Could you check a few things on this model? Use its own coordinates, in mm. Round coordinates to 2 decimals unless told otherwise and drop trailing zeros. Write each loop counter-clockwise with the first axis right and the second up, starting at its lowest first coordinate (ties: lowest second). Pieces come first, ordered by that corner, then holes. Notation, with made-up numbers: (32, 28) - (67, 28) arc R14 cw to (67, 35) - close; hole circle Ø11 at (-31, 29). An arc over 180 degrees is marked (long way). Write each question's results on one line, items separated by ' | '. Start each with the question number.
(1) Imagine slicing it at D-D on z = -28.5. Write out the boundary of the cut face in (x, y).
(2) Imagine slicing it at A-A on z = 0. Write out the boundary of the cut face in (x, y).
(3) Please list where these lines run through material, in increasing order: line 1 (X direction, y = 1.8, z = -24.5); line 2 (Z direction, x = -50, y = 2.05); line 3 (X direction, y = 1.2, z = 0). Write a range as [from, to].
(4) For P1, Ø3, axis at x = -100, z = -20, coming from the +Y side; P2, Ø0.9, axis at x = -119, y = 2, coming from the -Z side; P3, Ø1.5, axis at y = 1.5, z = -24.5, coming from the -X side, each with a flat end and sliding along its axis, tell me the tip position at first contact or that it passes through.
(5) Imagine slicing it at C-C on y = 0.65. State how many separate pieces and enclosed holes the cut face has, then the cut area to 3 significant figures.
(6) Imagine slicing it at B-B on x = 50. Write out the boundary of the cut face in (y, z).
(7) Thinking about a two-plate mould opening in X: for faces 1 (the flat face through (-2, 3, 15)), 2 (the cylindrical face through (-60, 2, 0)), 3 (the cylindrical face through (76, 1, 42)), which applies, +X half, -X half, draft (parallel to the pull), parting line (faces both ways), or undercut?
```python
from build123d import *

# Parameters (mm, degrees)
SKETCH1_W           = 220
SKETCH1_H           = 80
BOSS_EXTRUDE1_DEPTH = 3
SKETCH2_W           = 20
SKETCH2_H           = 20
SKETCH2_R           = 2
BOSS_EXTRUDE2_DEPTH = 3
FILLET1_R           = 5
SKETCH3_R           = 2
CUT_EXTRUDE1_DEPTH  = 3
SKETCH4_R           = 1.5
CUT_EXTRUDE2_DEPTH  = 3
SKETCH5_W           = 150
SKETCH5_H           = 22
BOSS_EXTRUDE3_DEPTH = 3
FILLET2_R           = 5
SKETCH6_R           = 10
CUT_EXTRUDE3_DEPTH  = 3
SKETCH7_R           = 2
CUT_EXTRUDE4_DEPTH  = 3


with BuildPart() as part:
    # Sketch1 → Boss-Extrude1 (new body)
    with BuildSketch(Plane(origin=(0, 0, 0), x_dir=(1, 0, 0), z_dir=(0, 1, 0))):
        Rectangle(SKETCH1_W, SKETCH1_H)
    extrude(amount=BOSS_EXTRUDE1_DEPTH)

    # Sketch2 → Boss-Extrude2 (add)
    with BuildSketch(Plane(origin=(0, 3, 0), x_dir=(1, 0, 0), z_dir=(0, 1, 0))):
        with Locations((-120, -30)):
            Rectangle(SKETCH2_W, SKETCH2_H)
        with Locations((-120, -32.5)):
            Circle(SKETCH2_R, mode=Mode.SUBTRACT)
    boss_extrude2 = extrude(amount=-BOSS_EXTRUDE2_DEPTH)

    # Mirror1: Boss-Extrude2 across plane
    add(boss_extrude2.mirror(Plane(origin=(0, 0, 0), x_dir=(0, 0, 1), z_dir=(1, 0, 0))))

    # Fillet1
    fillet1_edges = [part.edges().sort_by_distance(p)[0] for p in [
        (-110, 1.5, 20),
        (110, 1.5, 20),
    ]]
    fillet(fillet1_edges, radius=FILLET1_R)

    # Sketch3 → Cut-Extrude1 (cut)
    with BuildSketch(Plane(origin=(0, 3, 0), x_dir=(1, 0, 0), z_dir=(0, 1, 0))):
        with Locations((-100, 20)):
            Circle(SKETCH3_R)
        with Locations((100, 20)):
            Circle(SKETCH3_R)
    extrude(amount=-CUT_EXTRUDE1_DEPTH, mode=Mode.SUBTRACT)

    # Sketch4 → Cut-Extrude2 (cut)
    with BuildSketch(Plane(origin=(0, 3, 0), x_dir=(1, 0, 0), z_dir=(0, 1, 0))):
        with Locations((0, 24.5)):
            Circle(SKETCH4_R)
        with Locations((58, 24.5)):
            Circle(SKETCH4_R)
        with Locations((58, -24.5)):
            Circle(SKETCH4_R)
        with Locations((0, -24.5)):
            Circle(SKETCH4_R)
    extrude(amount=-CUT_EXTRUDE2_DEPTH, mode=Mode.SUBTRACT)

    # Sketch5 → Boss-Extrude3 (add)
    with BuildSketch(Plane(origin=(0, 3, 0), x_dir=(1, 0, 0), z_dir=(0, 1, 0))):
        with Locations((0, -40)):
            Rectangle(SKETCH5_W, SKETCH5_H)
    extrude(amount=-BOSS_EXTRUDE3_DEPTH)

    # Fillet2
    fillet2_edges = [part.edges().sort_by_distance(p)[0] for p in [
        (-75, 1.5, 40),
        (75, 1.5, 40),
    ]]
    fillet(fillet2_edges, radius=FILLET2_R)

    # Sketch6 → Cut-Extrude3 (cut)
    with BuildSketch(Plane(origin=(0, 3, 0), x_dir=(1, 0, 0), z_dir=(0, 1, 0))):
        with Locations((-50, 0)):
            Circle(SKETCH6_R)
        Circle(SKETCH6_R)
        with Locations((50, 0)):
            Circle(SKETCH6_R)
    extrude(amount=-CUT_EXTRUDE3_DEPTH, mode=Mode.SUBTRACT)

    # Sketch7 → Cut-Extrude4 (cut)
    with BuildSketch(Plane(origin=(0, 3, 0), x_dir=(1, 0, 0), z_dir=(0, 1, 0))):
        with Locations((-78, 20)):
            Circle(SKETCH7_R)
        with Locations((-44, 20)):
            Circle(SKETCH7_R)
        with Locations((-44, -20)):
            Circle(SKETCH7_R)
        with Locations((-78, -20)):
            Circle(SKETCH7_R)
    extrude(amount=-CUT_EXTRUDE4_DEPTH, mode=Mode.SUBTRACT)


solid = part.part
```
Response:
1) outline: (-110, 0) - (110, 0) - (110, 3) - (-110, 3) - close
2) outline: (-110, 0) - (-60, 0) - (-60, 3) - (-110, 3) - close; (-40, 0) - (-10, 0) - (-10, 3) - (-40, 3) - close; (10, 0) - (40, 0) - (40, 3) - (10, 3) - close; (60, 0) - (110, 0) - (110, 3) - (60, 3) - close
3) line 1: [-110, -1.5], [1.5, 56.5], [59.5, 110] | line 2: [-40, -10], [10, 51] | line 3: [-110, -60], [-40, -10], [10, 40], [60, 110]
4) P1: through | P2: z = 20 | P3: x = -110
5) separate pieces: 1 | enclosed holes: 15 | area: 19,000 mm²
6) outline: (0, -40) - (3, -40) - (3, -10) - (0, -10) - close; (0, 10) - (3, 10) - (3, 51) - (0, 51) - close
7) face 1: draft | face 2: undercut | face 3: +X half
